The model under review builds one solid part; all positions refer to its coordinate system, in mm. Face numbers are marked on the shaded views. A direction names the side the tool comes from. Coordinates: 2 decimals unless noted, no trailing zeros. Loops run counter-clockwise (first coordinate to the right, second up) from the corner with the lowest first, then second, coordinate; pieces in that order, holes last. Notation, with made-up numbers: M 6.5,65 L 35.5,65 A26 ccw 35.5,101 Z; hole C 25,77 d9. An arc over 180 degrees is marked long. Return JSON: item names as keys, results as strings.
```python
from build123d import *

# Parameters (mm, degrees)
FILLET1_R = 2.54


with BuildPart() as part:
    # Sketch1 → Revolve2 (revolve)
    with BuildSketch(Plane.XY, mode=Mode.PRIVATE) as revolve2_sk:
        Polygon((13.335, 0), (13.335, 33.02), (22.225, 52.07), (22.225, 63.5), (36.83, 63.5), (36.83, 38.1), (22.225, 38.1), (22.225, 0), align=None)
    revolve(revolve2_sk.sketch.rotate(Axis((0, 0, 0), (0, 1, 0)), 90), axis=Axis((0, 0, 0), (0, 1, 0)))

    # Fillet1
    fillet1_edges = [part.edges().sort_by_distance(p)[0] for p in [
        (0, 0, 22.225),
        (0, 33.02, 13.335),
        (0, 63.5, 22.225),
        (0, 63.5, 36.83),
        (0, 38.1, 36.83),
    ]]
    fillet(fillet1_edges, radius=FILLET1_R)


solid = part.part
```
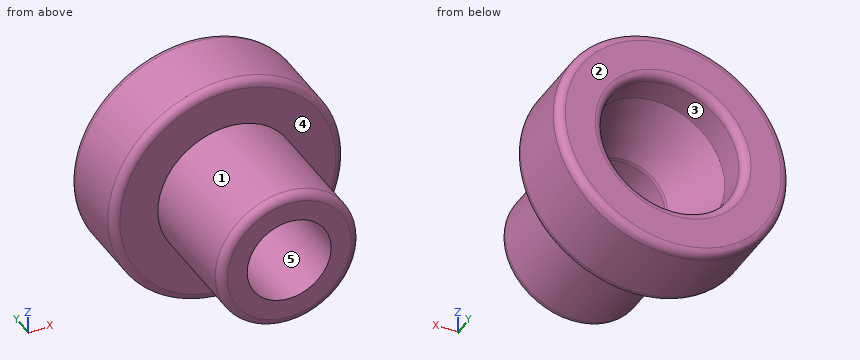
1. Add section B-B on y = 15.5. Give the boundary of the cut face in (x, z) (3 decimals), plus the area to 3 significant figures.
Check values:
{"outline": "C 0,0 d44.45; hole C 0,0 d26.67", "area": "993 mm²"}
2. The part is to be moulded in two halves that separate along Z. For the marked faces 1, 2 and 3, say which applies: released by +Z, released by -Z, zero draft, split by the parting line, or undercut.
Check values:
{"face 1": "split by the parting line", "face 2": "zero draft", "face 3": "undercut"}
3. Machinability: for the marked faces 4 and 5, which of the approach directions +Z, -Z, +X, -X, +Y, -Y give a long, thin tool a straight path to every point of the face, cutting with its end or side? Answer none if there is none.
Check values:
{"face 4": "-Y", "face 5": "+Y, -Y"}
4. Add section A-A on y = 48. Give the boundary of the cut face in (x, z), plus the area to 3 significant figures.
Check values:
{"outline": "C 0,0 d73.66; hole C 0,0 d40.65", "area": "2,960 mm²"}
5. Insertion check: pin 1 Ø1.5 at (y, z) = (43, 28.5) entering from -X; pin 2 Ø2 at (y, z) = (35.5, 27) entering from +X; pin 3 Ø2 at (x, y) = (4.5, 56.5) entering from -Z; pin 4 Ø1.5 at (x, z) = (-27, 24) entering from -Y. Each pin has a flat end and moves straight along its axis. Give the tip position at first contact, or say it passes through.
Check values:
{"pin 1": "x = -24.22", "pin 2": "through", "pin 3": "z = -36.66", "pin 4": "y = 38.34"}
6. To check wall thickness, follow line 1 (X direction, y = 15.5, z = 0) (3 decimals); line 2 (X direction, y = 57, z = 0) (3 decimals); line 3 (Y direction, x = -33.5, z = 3.5). State the ranges of each line that lie inside material, in increasing order.
Check values:
{"line 1": "-22.225 to -13.335, 13.335 to 22.225", "line 2": "-36.83 to -22.225, 22.225 to 36.83", "line 3": "38.1 to 63.5"}
